Could you check a few things on this model? Use its own coordinates, in mm. Give positions to 0.01 mm unless a question says otherwise; leave off trailing zeros. Loops run counter-clockwise (first coordinate to the right, second up) from the corner with the lowest first, then second, coordinate; pieces in that order, holes last.
1. Imagine slicing it at A-A (x = 62). List the corners of the cut face in (y, z) for me.
2. Imagine slicing it at B-B (z = 2). Count the separate pieces of the cut face and the enclosed holes in it, plus the area to 3 significant figures.
3. I need wall thicknesses on line 1 along Y through (x, z) = (-101.6, 4.5); line 2 along X through (y, z) = (220.98, 3.5) (3 decimals); line 3 along Y through (x, z) = (115, 1.5). Which ranges of each line are inside material? Lowest first, please.
4. Thinking about a two-plate mould opening in Y: for faces 1 (the cylindrical face through (-133.97, 178.15, 3.13)), 2 (the flat face through (33, 146, 6.35)), 3 (the cylindrical face through (175.94, 237.686, 3.131)), which applies, +Y half, -Y half, draft (parallel to the pull), parting line (faces both ways), or undercut?
5. Imagine slicing it at C-C (x = -66). List the corners of the cut face in (y, z) for me, plus the area to 3 significant figures.
6. Imagine slicing it at D-D (y = -43). List the corners of the cut face in (x, z) for me.
7. For P1, Ø15.5, axis at x = -101.31, y = 210.82, coming from the +Z side (1 decimal); P2, Ø3, axis at y = 53, z = 4, coming from the -X side; P3, Ø2, axis at x = 142, z = 1, coming from the -Y side; P4, Ø1, axis at y = -43, z = 4, coming from the -X side, each with a flat end and sliding along its axis, tell me the tip position at first contact or that it passes through.
```python
from build123d import *

# Parameters (mm, degrees)
SKETCH1_R           = 14.2875
SKETCH1_R_2         = 3.175
SKETCH1_R_3         = 9.652
SKETCH1_R_4         = 2.032
BOSS_EXTRUDE3_DEPTH = 6.35


with BuildPart() as part:
    # Sketch1 → Boss-Extrude3 (new body)
    with BuildSketch(Plane.XY):
        with BuildLine():
            Line((0, 1.972692091), (0, 160.02))
            ThreePointArc((0, 160.02), (-3.719743879, 169.000256121), (-12.7, 172.72))
            Line((-12.7, 172.72), (-101.6, 172.72))
            Line((-101.6, 172.72), (-120.65, 172.72))
            ThreePointArc((-120.65, 172.72), (-134.120384182, 178.299615818), (-139.7, 191.77))
            Line((-139.7, 191.77), (-139.7, 229.87))
            ThreePointArc((-139.7, 229.87), (-134.120384182, 243.340384182), (-120.65, 248.92))
            Line((-120.65, 248.92), (-101.6, 248.92))
            Line((-101.6, 248.92), (0, 248.92))
            Line((0, 248.92), (4.7625, 248.92))
            Line((4.7625, 248.92), (198.4375, 248.92))
            ThreePointArc((198.4375, 248.92), (201.805096045, 247.525096045), (203.2, 244.1575))
            Line((203.2, 244.1575), (203.2, 203.159397936))
            ThreePointArc((203.2, 203.159397936), (201.73893916, 199.726919863), (198.252218068, 198.400503437))
            ThreePointArc((198.252218068, 198.400503437), (55.900468813, 87.207475286), (141.92702513, -71.623698082))
            ThreePointArc((141.92702513, -71.623698082), (144.874483412, -76.941407786), (140.194292932, -80.82230509))
            Line((140.194292932, -80.82230509), (82.79499718, -80.82230509))
            ThreePointArc((82.79499718, -80.82230509), (80.972467334, -80.459781363), (79.427401135, -79.427401135))
            Line((79.427401135, -79.427401135), (1.394903955, -1.394903955))
            ThreePointArc((1.394903955, -1.394903955), (0.362523726, 0.150162244), (0, 1.972692091))
        make_face()
        with Locations((177.8, 223.52)):
            Circle(SKETCH1_R, mode=Mode.SUBTRACT)
        with Locations((132.256792932, -73.51980509)):
            Circle(SKETCH1_R_2, mode=Mode.SUBTRACT)
        with Locations((81.456792932, -52.06873783)):
            Circle(SKETCH1_R_2, mode=Mode.SUBTRACT)
        with Locations((25.4, 220.98)):
            Circle(SKETCH1_R_2, mode=Mode.SUBTRACT)
        with Locations((-101.311264174, 210.821094089)):
            Circle(SKETCH1_R_3, mode=Mode.SUBTRACT)
        with Locations((-75.911264174, 210.821094089)):
            Circle(SKETCH1_R_4, mode=Mode.SUBTRACT)
        with Locations((-126.711264174, 210.821094089)):
            Circle(SKETCH1_R_4, mode=Mode.SUBTRACT)
        with Locations((-101.6, 236.221094089)):
            Circle(SKETCH1_R_4, mode=Mode.SUBTRACT)
        with Locations((-101.6, 185.421094089)):
            Circle(SKETCH1_R_4, mode=Mode.SUBTRACT)
    extrude(amount=BOSS_EXTRUDE3_DEPTH)


solid = part.part
```
Derived:
1. outline: (-62, 0) - (9.17, 0) - (9.17, 6.35) - (-62, 6.35) - close; (108.13, 0) - (248.92, 0) - (248.92, 6.35) - (108.13, 6.35) - close
2. separate pieces: 1
2. enclosed holes: 9
2. area: 39,400 mm2
3. line 1: y = 172.72 to 183.39, 187.45 to 201.17, 220.47 to 234.19, 238.25 to 248.92
3. line 2: x = -139.7 to 22.225, 28.575 to 163.74, 191.86 to 203.2
3. line 3: y = -80.82 to -57.56, 174.86 to 248.92
4. face 1: -Y half
4. face 2: draft
4. face 3: undercut
5. outline: (172.72, 0) - (248.92, 0) - (248.92, 6.35) - (172.72, 6.35) - close
5. area: 484 mm2
6. outline: (43, 0) - (96.75, 0) - (96.75, 6.35) - (43, 6.35) - close
7. P1: passes through
7. P2: stops at x = 0
7. P3: stops at y = -80.75
7. P4: stops at x = 42.5
